Geometry check sheet. Reference: drawing and pictorial views, mm from the part's lowest x, y, z. Give positions to 0.01 mm unless a question says otherwise; leave off trailing zeros. Order: outer loops, then holes, each group sorted by start corner. A loop starts at its lowest first (then second) coordinate and runs counter-clockwise, first axis right, second up.
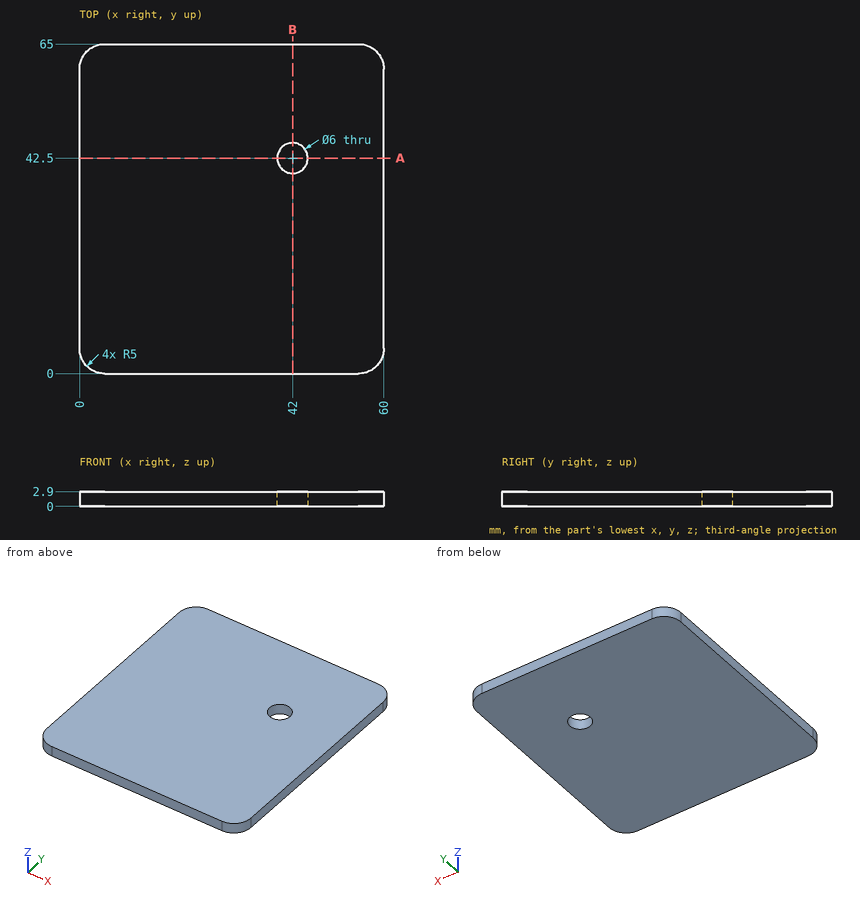
(1) Material ranges on L1, parallel to Y at x = 42, z = 1.15; L2, parallel to X at y = 43, z = 2.35; L3, parallel to Y at x = 56, z = 1.05, recorded low to high.
Response values:
L1: y = 0 to 39.5, 45.5 to 65
L2: x = 0 to 39.04, 44.96 to 60
L3: y = 0.1 to 64.9
(2) Cross-section at B-B on x = 42. Enter the section's corners in (y, z).
Response values:
outline: (0, 0) - (39.5, 0) - (39.5, 2.9) - (0, 2.9) - close; (45.5, 0) - (65, 0) - (65, 2.9) - (45.5, 2.9) - close
(3) Cross-section at A-A on y = 42.5. Enter the section's corners in (x, z), then the cut area to 3 significant figures.
Response values:
outline: (0, 0) - (39, 0) - (39, 2.9) - (0, 2.9) - close; (45, 0) - (60, 0) - (60, 2.9) - (45, 2.9) - close
area: 157 mm2
